Here's how the part is built. I have some questions about the finished solid (model axes, mm). A direction names the side the tool comes from. Round coordinates to 2 decimals unless told otherwise and drop trailing zeros. Write each loop counter-clockwise with the first axis right and the second up, starting at its lowest first coordinate (ties: lowest second). Pieces come first, ordered by that corner, then holes. Notation, with made-up numbers: (-16, 16) - (11, 16) arc R17 cw to (11, 37) - close; hole circle Ø2 at (-32, 7.25). An arc over 180 degrees is marked (long way). Use one line per item in the form item = value. Start each with the question number.
1. If I drill on line 1 along Y through (x, z) = (1.6, 146); line 2 along Y through (x, z) = (0.8, 25); line 3 along Y through (x, z) = (1.2, 159.5), over which ranges is the centre line in solid material (lowest first)?
2. We'd pull the mould along Z, two halves only. Please class faces 1 (the flat face through (1.039, 62.784, 157.8)), 2 (the flat face through (0, 24, 98)), 3 (the cylindrical face through (0.2, 58, 147)): +Z half, -Z half, draft (parallel to the pull), parting line (faces both ways), or undercut.
3. I want a section at A-A, the plane y = 88. List the corners of the cut face in (x, z) for me, plus the area to 3 significant figures.
4. Which directions (+Z, -Z, +X, -X, +Y, -Y) give clear straight access to the entire face, cutting with the end or side of a thin tool? Please do faces 4 (the flat face through (1.039, 46.57, 145.724)), 5 (the flat face through (1.039, 15.524, 14.739)), 6 (the flat face through (1.43, 31.88, 90.32)).
5. Will these pins go through, and if not, where does the flat tip stop? pin 1 (1.1 mm diameter, centred on x = 1.5, y = 85, fed in from -Z); pin 2 (1.1 mm diameter, centred on x = 0.5, z = 118.5, fed in from +Y); pin 3 (1 mm diameter, centred on x = 1, z = 22, fed in from +Y).
6. I want a section at B-B, the plane x = 1.4. State how many separate pieces and enclosed holes the cut face has, plus the area to 3 significant figures.
```python
from build123d import *

# Parameters (mm, degrees)
F0_W     = 5.08
F0_H     = 2.54
F1_DEPTH = 2.1082
F2_R     = 0.762


with BuildPart() as f1:
    # F0 (on Right) → F1 (new body)
    with BuildSketch(Plane.YZ):
        with BuildLine():
            Line((0, 162.0091375), (0, 0))
            Line((0, 0), (12.335197777, 0))
            Line((12.335197777, 0), (18.8042013144, 29.896105485))
            Line((18.8042013144, 29.896105485), (30.5493542935, 2.3257501254))
            Line((30.5493542935, 2.3257501254), (31.5401391658, 0))
            Line((31.5401391658, 0), (31.5707651968, 0))
            Line((31.5707651968, 0), (40.8442968098, 0))
            Line((40.8442968098, 0), (20.5594925834, 47.616175108))
            Line((20.5594925834, 47.616175108), (39.5771112022, 135.5049402038))
            Line((39.5771112022, 135.5049402038), (73.5248959406, 160.7899383022))
            Line((73.5248959406, 160.7899383022), (100.203, 160.7899383022))
            Line((100.203, 160.7899383022), (100.203, 162.0091375))
            Line((100.203, 162.0091375), (82.1398573303, 162.0091375))
            ThreePointArc((82.1398573303, 162.0091375), (80.3438061061, 162.7530862758), (79.5998573303, 164.5491375))
            Line((79.5998573303, 164.5491375), (79.5998573303, 169.3418))
            Line((79.5998573303, 169.3418), (70.6874244764, 169.3418))
            Line((70.6874244764, 169.3418), (70.6874244764, 165.8480664454))
            Line((70.6874244764, 165.8480664454), (70.6874244764, 164.5491375))
            ThreePointArc((70.6874244764, 164.5491375), (70.0510915867, 162.8675752701), (68.4609272063, 162.0285589874))
            ThreePointArc((68.4609272063, 162.0285589874), (68.3044763435, 162.0139975214), (68.1474244764, 162.0091375))
            Line((68.1474244764, 162.0091375), (0, 162.0091375))
        make_face()
        Polygon((21.4843682503, 35.8535070154), (23.4753466245, 31.1799211209), (21.1385536773, 30.1844319338), (19.147575303, 34.8580178283), align=None, mode=Mode.SUBTRACT)
        Polygon((25.8665425285, 25.5668719827), (27.8575209028, 20.8932860882), (25.5207279555, 19.8977969011), (23.5297495813, 24.5713827956), align=None, mode=Mode.SUBTRACT)
        with BuildLine():
            Line((12.3986134924, 50.3752630702), (11.6175919588, 46.7658196656))
            Line((11.6175919588, 46.7658196656), (10.5918, 46.7658196656))
            Line((10.5918, 46.7658196656), (10.5918, 158.7579375))
            Line((10.5918, 158.7579375), (35.8507619547, 158.7579375))
            Line((35.8507619547, 158.7579375), (31.8897708968, 140.4524587956))
            Line((31.8897708968, 140.4524587956), (31.1087493632, 136.8430153909))
            Line((31.1087493632, 136.8430153909), (35.5475592049, 135.882533211))
            ThreePointArc((35.5475592049, 135.882533211), (37.1456481821, 134.7755682604), (37.4929253116, 132.8628062845))
            Line((37.4929253116, 132.8628062845), (29.5595533377, 96.1992113407))
            ThreePointArc((29.5595533377, 96.1992113407), (28.452588387, 94.6011223635), (26.5398264112, 94.2538452339))
            Line((26.5398264112, 94.2538452339), (22.1010165695, 95.2143274138))
            Line((22.1010165695, 95.2143274138), (21.7536814278, 93.6091392306))
            Line((21.7536814278, 93.6091392306), (21.4063462861, 92.0039510473))
            Line((21.4063462861, 92.0039510473), (25.8451561277, 91.0434688674))
            ThreePointArc((25.8451561277, 91.0434688674), (27.4432451049, 89.9365039168), (27.7905222345, 88.0237419409))
            Line((27.7905222345, 88.0237419409), (19.8571502605, 51.3601469971))
            ThreePointArc((19.8571502605, 51.3601469971), (18.7501853099, 49.7620580199), (16.837423334, 49.4147808903))
            Line((16.837423334, 49.4147808903), (12.3986134924, 50.3752630702))
        make_face(mode=Mode.SUBTRACT)
        Polygon((47.0613097153, 149.2568137468), (48.5785484084, 147.2197602993), (44.5044415132, 144.1852829132), (42.9872028202, 146.2223363607), align=None, mode=Mode.SUBTRACT)
        Polygon((44.8088104432, 150.074821282), (46.6876875952, 158.7579375), (56.4668125154, 158.7579375), align=None, mode=Mode.SUBTRACT)
        Polygon((63.2751536106, 161.3332132886), (64.7923923036, 159.296159841), (60.7182854085, 156.2616824549), (59.2010467154, 158.2987359025), align=None, mode=Mode.SUBTRACT)
        with BuildLine():
            Line((0, 164.5491375), (0, 162.0091375))
            Line((0, 162.0091375), (68.1474244764, 162.0091375))
            ThreePointArc((68.1474244764, 162.0091375), (68.3044763435, 162.0139975214), (68.4609272063, 162.0285589874))
            Line((68.4609272063, 162.0285589874), (69.6856973646, 162.9407926238))
            Line((69.6856973646, 162.9407926238), (68.1474244764, 165.0060867035))
            Line((68.1474244764, 165.0060867035), (68.1474244764, 164.5491375))
            Line((68.1474244764, 164.5491375), (55.1748093832, 164.5491375))
            Line((55.1748093832, 164.5491375), (50.0948093832, 164.5491375))
            Line((50.0948093832, 164.5491375), (10.3999171089, 164.5491375))
            Line((10.3999171089, 164.5491375), (5.3199171089, 164.5491375))
            Line((5.3199171089, 164.5491375), (0, 164.5491375))
        make_face()
        Polygon((0, 169.3418), (0, 164.5491375), (5.3199171089, 164.5491375), (5.3199171089, 167.0891375), (10.3999171089, 167.0891375), (10.3999171089, 164.5491375), (50.0948093832, 164.5491375), (50.0948093832, 167.0891375), (55.1748093832, 167.0891375), (55.1748093832, 164.5491375), (68.1474244764, 164.5491375), (68.1474244764, 165.0060867035), (68.1474244764, 169.3418), align=None)
        with Locations((7.8599171089, 165.8191375)):
            Rectangle(F0_W, F0_H)
        with BuildLine():
            Line((69.6856973646, 162.9407926238), (68.4609272063, 162.0285589874))
            ThreePointArc((68.4609272063, 162.0285589874), (70.0510915867, 162.8675752701), (70.6874244764, 164.5491375))
            Line((70.6874244764, 164.5491375), (70.6874244764, 165.8480664454))
            Line((70.6874244764, 165.8480664454), (70.6874244764, 169.3418))
            Line((70.6874244764, 169.3418), (68.1474244764, 169.3418))
            Line((68.1474244764, 169.3418), (68.1474244764, 165.0060867035))
            Line((68.1474244764, 165.0060867035), (69.6856973646, 162.9407926238))
        make_face()
        with Locations((52.6348093832, 165.8191375)):
            Rectangle(F0_W, F0_H)
        with BuildLine():
            Line((20.5594925834, 47.616175108), (40.8442968098, 0))
            Line((40.8442968098, 0), (43.053, 0))
            Line((43.053, 0), (23.4736756901, 45.9601445708))
            ThreePointArc((23.4736756901, 45.9601445708), (22.9941781878, 47.847708452), (23.1092917667, 49.7918185633))
            Line((23.1092917667, 49.7918185633), (40.8984089502, 132.0031391675))
            ThreePointArc((40.8984089502, 132.0031391675), (41.765080018, 134.0967787378), (43.3116785091, 135.7528217618))
            Line((43.3116785091, 135.7528217618), (72.5103326221, 157.500571119))
            ThreePointArc((72.5103326221, 157.500571119), (74.3053957564, 158.4354047741), (76.3034293547, 158.7579375))
            Line((76.3034293547, 158.7579375), (100.203, 158.7579375))
            Line((100.203, 158.7579375), (100.203, 160.7899383022))
            Line((100.203, 160.7899383022), (73.5248959406, 160.7899383022))
            Line((73.5248959406, 160.7899383022), (39.5771112022, 135.5049402038))
            Line((39.5771112022, 135.5049402038), (20.5594925834, 47.616175108))
        make_face()
        with BuildLine():
            Line((82.1398573303, 169.3418), (79.5998573303, 169.3418))
            Line((79.5998573303, 169.3418), (79.5998573303, 164.5491375))
            ThreePointArc((79.5998573303, 164.5491375), (80.3438061061, 162.7530862758), (82.1398573303, 162.0091375))
            Line((82.1398573303, 162.0091375), (100.203, 162.0091375))
            Line((100.203, 162.0091375), (100.203, 164.5491375))
            Line((100.203, 164.5491375), (89.6502663064, 164.5491375))
            Line((89.6502663064, 164.5491375), (84.5702663064, 164.5491375))
            Line((84.5702663064, 164.5491375), (82.1398573303, 164.5491375))
            Line((82.1398573303, 164.5491375), (82.1398573303, 169.3418))
        make_face()
        Polygon((100.203, 169.3418), (82.1398573303, 169.3418), (82.1398573303, 164.5491375), (84.5702663064, 164.5491375), (84.5702663064, 167.0891375), (89.6502663064, 167.0891375), (89.6502663064, 164.5491375), (100.203, 164.5491375), align=None)
        with BuildLine():
            Line((12.9357939022, 52.8578095868), (12.3986134924, 50.3752630702))
            Line((12.3986134924, 50.3752630702), (16.837423334, 49.4147808903))
            ThreePointArc((16.837423334, 49.4147808903), (18.7501853099, 49.7620580199), (19.8571502605, 51.3601469971))
            Line((19.8571502605, 51.3601469971), (27.7905222345, 88.0237419409))
            ThreePointArc((27.7905222345, 88.0237419409), (27.4432451049, 89.9365039168), (25.8451561277, 91.0434688674))
            Line((25.8451561277, 91.0434688674), (21.4063462861, 92.0039510473))
            Line((21.4063462861, 92.0039510473), (20.8691658762, 89.5214045307))
            Line((20.8691658762, 89.5214045307), (25.3079757178, 88.5609223508))
            Line((25.3079757178, 88.5609223508), (24.0175885553, 82.5974767434))
            Line((24.0175885553, 82.5974767434), (22.9432277355, 77.6323837102))
            Line((22.9432277355, 77.6323837102), (19.7419229759, 62.8377489213))
            Line((19.7419229759, 62.8377489213), (18.6675621562, 57.872655888))
            Line((18.6675621562, 57.872655888), (17.3746037439, 51.8973274069))
            Line((17.3746037439, 51.8973274069), (12.9357939022, 52.8578095868))
        make_face()
        Polygon((20.8691658762, 89.5214045307), (12.9357939022, 52.8578095868), (17.3746037439, 51.8973274069), (18.6675621562, 57.872655888), (16.1850156395, 58.4098362979), (17.2593764593, 63.3749293312), (19.7419229759, 62.8377489213), (22.9432277355, 77.6323837102), (20.4606812189, 78.16956412), (21.5350420386, 83.1346571533), (24.0175885553, 82.5974767434), (25.3079757178, 88.5609223508), align=None)
        with BuildLine():
            Line((35.5475592049, 135.882533211), (31.1087493632, 136.8430153909))
            Line((31.1087493632, 136.8430153909), (30.5715689534, 134.3604688743))
            Line((30.5715689534, 134.3604688743), (35.010378795, 133.3999866944))
            Line((35.010378795, 133.3999866944), (33.7174203827, 127.4246582133))
            Line((33.7174203827, 127.4246582133), (32.643059563, 122.45956518))
            Line((32.643059563, 122.45956518), (29.4417548033, 107.6649303911))
            Line((29.4417548033, 107.6649303911), (28.3673939836, 102.6998373579))
            Line((28.3673939836, 102.6998373579), (27.077006821, 96.7363917505))
            Line((27.077006821, 96.7363917505), (22.6381969794, 97.6968739305))
            Line((22.6381969794, 97.6968739305), (22.1010165695, 95.2143274138))
            Line((22.1010165695, 95.2143274138), (26.5398264112, 94.2538452339))
            ThreePointArc((26.5398264112, 94.2538452339), (28.452588387, 94.6011223635), (29.5595533377, 96.1992113407))
            Line((29.5595533377, 96.1992113407), (37.4929253116, 132.8628062845))
            ThreePointArc((37.4929253116, 132.8628062845), (37.1456481821, 134.7755682604), (35.5475592049, 135.882533211))
        make_face()
        Polygon((35.010378795, 133.3999866944), (30.5715689534, 134.3604688743), (22.6381969794, 97.6968739305), (27.077006821, 96.7363917505), (28.3673939836, 102.6998373579), (25.884847467, 103.2370177677), (26.9592082867, 108.202110801), (29.4417548033, 107.6649303911), (32.643059563, 122.45956518), (30.1605130463, 122.9967455899), (31.2348738661, 127.9618386231), (33.7174203827, 127.4246582133), align=None)
    extrude(amount=F1_DEPTH)

    # F2
    f2_edges = [f1.edges().sort_by_distance(p)[0] for p in [
        (0, 57.911006, 146.626696),
        (0, 33.263338, 22.980072),
        (0, 22.994178, 47.847708),
        (0, 32.00385, 90.897479),
        (0, 41.76508, 134.096779),
        (0, 74.305396, 158.435405),
        (0, 88.253215, 158.757937),
    ]]
    fillet(f2_edges, radius=F2_R)


solid = f1.part
```
Model answer:
q1.line_1 = 0 to 10.59, 33.09 to 43.15, 46.94 to 57.07
q1.line_2 = 0 to 17.74, 20.89 to 24.54, 26.11 to 32.4
q1.line_3 = 0 to 60.81, 64.64 to 100.2
q2.face_1 = undercut
q2.face_2 = draft
q2.face_3 = -Z half
q3.outline = (0, 159.52) arc R0.76 ccw to (0.76, 158.76) - (2.11, 158.76) - (2.11, 164.55) - (0, 164.55) - close; (0, 167.09) - (2.11, 167.09) - (2.11, 169.34) - (0, 169.34) - close
q3.area = 16.8 mm2
q4.face_4 = +X, -X
q4.face_5 = -Z, +X, -X
q4.face_6 = +X, -X, +Y
q5.pin_1 = 158.76
q5.pin_2 = 38.08
q5.pin_3 = 33.89
q6.separate_pieces = 1
q6.enclosed_holes = 11
q6.area = 4,900 mm2
